from build123d import *

# Parameters (mm, degrees)
F3_R     = 8.751672
F4_DEPTH = 25
F5_R     = 5


with BuildPart() as f2:
    # F0 (on Right) → F2 (revolve)
    with BuildSketch(Plane.YZ):
        Polygon((10, 60.288332), (0, 60.288332), (0, 57.74051), (6.906209, 57.74051), (6.906209, 50.288332), (15.09565, 42.280882), (15.09565, 2.780263), (0, 2.780263), (0, 0), (17.2795, 0), (17.2795, 42.826841), (10, 50.288332), align=None)
    revolve(axis=Axis((0, 0, 30.372418), (0, 0, 1)))

    # F3 (on face) → F4 (cut)
    with BuildSketch(Plane.XY.offset(60.288332)):
        Circle(F3_R)
    extrude(amount=-F4_DEPTH, mode=Mode.SUBTRACT)

    # F5
    f5_edges = [f2.edges().sort_by_distance(p)[0] for p in [
        (0, -10, 50.288332),
        (0, -17.2795, 42.826841),
        (0, -17.2795, 0),
    ]]
    fillet(f5_edges, radius=F5_R)


solid = f2.part
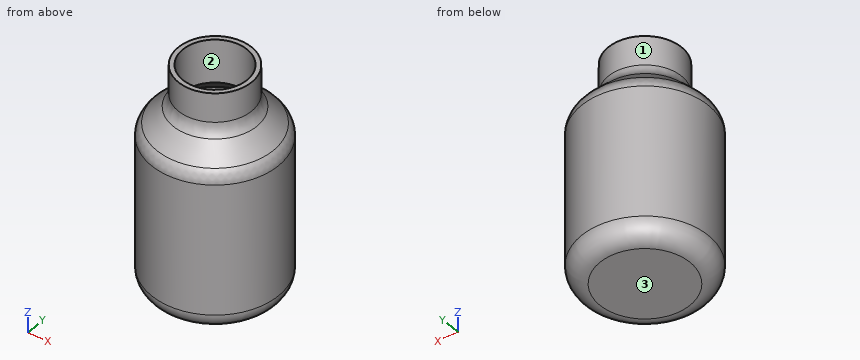
Input: part model. Units: mm. Frame: model coordinates. Face numbers are marked on the shaded views. Round coordinates to 2 decimals unless told otherwise and drop trailing zeros. Write each loop counter-clockwise with the first axis right and the second up, starting at its lowest first coordinate (ties: lowest second). Pieces come first, ordered by that corner, then holes.
1) Ray query, L1, parallel to X at y = 0, z = 20; L2, parallel to X at y = 0, z = 56. Return the intervals inside material, ascending.
2) Draft query along X for the marked faces 1, 2 and 3. Return one class per face: pulls with the +X half, pulls with the -X half, needs draft (parallel to the pull), parting line crosses it, or undercut.
3) Cut plane A-A (z = 11). Return the cut outline in (x, y), then the cut area to 3 significant figures.
4) Contact query for flat-ended pins moving along their axis: P1, Ø1, axis at x = -5.5, y = 11.5, coming from the +Z side; P2, Ø4, axis at x = -3, y = -0.5, coming from the +Z side; P3, Ø1, axis at y = -9, z = 48, coming from the -X side. Output: stop coordinate, or through.
Geometry says:
1. L1: x = -17.28 to -15.1, 15.1 to 17.28
1. L2: x = -10 to -8.75, 8.75 to 10
2. face 1: parting line crosses it
2. face 2: undercut
2. face 3: needs draft
3. outline: circle Ø34.56 at (0, 0); hole circle Ø30.19 at (0, 0)
3. area: 222 mm2
4. P1: stops at z = 47.98
4. P2: stops at z = 2.78
4. P3: stops at x = -9.15
